Geometry: final body of the model. Coordinates: model frame, mm. A direction names the side the tool comes from. Give positions to 0.01 mm unless a question says otherwise; leave off trailing zeros. Order: outer loops, then holes, each group sorted by start corner. A loop starts at its lowest first (then second) coordinate and runs counter-clockwise, first axis right, second up. Notation, with made-up numbers: (36.25, -31.75) - (84.25, -31.75) arc R19 ccw to (84.25, -23.75) - close; hole circle Ø6 at (-14.5, 5.5). An arc over 180 degrees is marked (long way). Use one line per item in the form item = value.
from build123d import *

# Parameters (mm, degrees)
EXTRUDE_1_DEPTH     = 9
CUT_EXTRUDE_START   = 7.5
CUT_EXTRUDE_1_DEPTH = 142.076331988
CUT_EXTRUDE_START_2 = 8
CUT_EXTRUDE_2_DEPTH = 141.576331988
CUT_EXTRUDE_START_3 = 4.5
CUT_EXTRUDE_3_DEPTH = 145.076331988
CHAMFER_1_SIZE      = 1


# Read off the part's stored shape, not the designer's step: M22 机械螺纹 螺柱1
with BuildPart() as part:
    # 草图1 → 旋转1 (revolve)
    with BuildSketch(Plane.XY, mode=Mode.PRIVATE) as revolve_1_sk:
        Polygon((0, 0), (0, 8.5), (3.9, 8.5), (3.9, 8.1), (5, 8.1), (5, 8.5), (17, 8.5), (17, 12), (34, 12), (34, 17.5), (40, 17.5), (40, 12.5), (55, 12.5), (55, 11), (97, 11), (97, 8.5), (109, 8.5), (109, 7.5), (124, 7.5), (124, 0), align=None)
    revolve(revolve_1_sk.sketch.rotate(Axis((0, 0, 0), (1, 0, 0)), 90), axis=Axis((0, 0, 0), (1, 0, 0)))

    # 草图2 → 凸台-拉伸1 (add)
    with BuildSketch(Plane.ZY.offset(-34)):
        with BuildLine():
            ThreePointArc((1.769346299, -11.868842137), (-12, 0), (1.769346299, 11.868842137))
            ThreePointArc((1.769346299, 11.868842137), (-17.516638735, 20.354713861), (-29.814759189, 37.463643428))
            ThreePointArc((-29.814759189, 37.463643428), (-31.910579937, 39.994896928), (-35.125, 40.678426408))
            ThreePointArc((-35.125, 40.678426408), (-71, 0), (-35.125, -40.678426408))
            ThreePointArc((-35.125, -40.678426408), (-31.910579937, -39.994896928), (-29.814759189, -37.463643428))
            ThreePointArc((-29.814759189, -37.463643428), (-17.516638735, -20.354713861), (1.769346299, -11.868842137))
        make_face()
    extrude(amount=EXTRUDE_1_DEPTH)

    # 草图3 → 切除-拉伸1 (cut, through all)
    with BuildSketch(Plane.XY.offset(CUT_EXTRUDE_START)):
        with BuildLine():
            Line((59, 3), (71, 3))
            ThreePointArc((71, 3), (74, 0), (71, -3))
            Line((71, -3), (59, -3))
            ThreePointArc((59, -3), (56, 0), (59, 3))
        make_face()
    extrude(amount=CUT_EXTRUDE_1_DEPTH, mode=Mode.SUBTRACT)

    # M22 机械螺纹 螺柱1 outline → M22 机械螺纹 螺柱1 (revolve, cut)
    with BuildSketch(Plane.YX):
        Polygon((11, 97), (9.647, 97), (11, 95.647), align=None)
    revolve(axis=Axis((0, 0, 0), (1, 0, 0)), mode=Mode.SUBTRACT)

    # 草图4 → 切除-拉伸2 (cut, through all)
    with BuildSketch(Plane.XY.offset(CUT_EXTRUDE_START_2)):
        with BuildLine():
            Line((81, 2.5), (110.572522736, 2.5))
            ThreePointArc((110.572522736, 2.5), (113.072522736, 0), (110.572522736, -2.5))
            Line((110.572522736, -2.5), (81, -2.5))
            ThreePointArc((81, -2.5), (78.5, 0), (81, 2.5))
        make_face()
    extrude(amount=CUT_EXTRUDE_2_DEPTH, mode=Mode.SUBTRACT)

    # 草图6 → 切除-拉伸3 (cut, through all)
    with BuildSketch(Plane.XY.offset(CUT_EXTRUDE_START_3)):
        with BuildLine():
            Line((111.5, 2.5), (120.5, 2.5))
            ThreePointArc((120.5, 2.5), (123, 0), (120.5, -2.5))
            Line((120.5, -2.5), (111.5, -2.5))
            ThreePointArc((111.5, -2.5), (109, 0), (111.5, 2.5))
        make_face()
    extrude(amount=CUT_EXTRUDE_3_DEPTH, mode=Mode.SUBTRACT)

    # 倒角1
    chamfer_1_edges = [part.edges().sort_by_distance(p)[0] for p in [
        (124, 0, -7.5),
        (0, 0, -8.5),
    ]]
    chamfer(chamfer_1_edges, length=CHAMFER_1_SIZE)


solid = part.part
(1) Ray query, line 1 along X through (y, z) = (12.5, -60); line 2 along Z through (x, y) = (46, 6); line 3 along Y through (x, z) = (57, 8). Return the intervals inside material, ascending.
Computed values:
line_1 = 25 to 34
line_2 = -10.97 to 10.97
line_3 = -7.55 to -2.24, 2.24 to 7.55
(2) Cut plane B-B on y = 19.5. Output: boundary loops of the cut face in (x, z), plus the area to 3 significant figures.
Computed values:
outline = (25, -66.07) - (34, -66.07) - (34, -16.42) - (25, -16.42) - close
area = 447 mm²
(3) Cut plane C-C on x = 21. Output: boundary loops of the cut face in (y, z).
Computed values:
outline = circle Ø24 at (0, 0)
(4) Contact query for flat-ended pins moving along their axis: pin 1 Ø6.5 at (x, y) = (63.5, -1) entering from +Z; pin 2 Ø12 at (x, z) = (106, 4) entering from +Y; pin 3 Ø0.8 at (x, z) = (89, 9) entering from -Y; pin 4 Ø13 at (y, z) = (-5.5, 2.5) entering from -X. Output: stop coordinate, or through.
Computed values:
pin_1 = 10.58
pin_2 = 8.5
pin_3 = -6.86
pin_4 = 0
(5) Reachability of faces 1 (the face through (34, -0.1, 12.2)), 2 (the face through (23.73, 4.596, 11.085)), 3 (the face through (123, 0, 6)), 4 (the face through (97, 4, -8)), 5 (the face through (29.563, -20.544, -17.748)) from +Z, -Z, +X, -X, +Y, -Y: full face, straight path, thin tool, end or side. Return the list, or none.
Computed values:
face_1 = +Z, -X
face_2 = -X
face_3 = +Z
face_4 = +X
face_5 = +Z, -X, -Y
(6) Pull-direction query (Y, two-part tool) for faces 6 (the face through (94, 0, 8)), 7 (the face through (47.605, -3.755, 11.923)), 8 (the face through (17, -8.2, 2.8)); classes: released by +Y, released by -Y, zero draft, split by the parting line, or undercut.
Computed values:
face_6 = undercut
face_7 = split by the parting line
face_8 = zero draft
(7) Cut plane A-A on x = 103. Output: boundary loops of the cut face in (y, z).
Computed values:
outline = (-2.5, 8) - (-2.5, 8.12) arc R8.5 ccw (long way) to (2.5, 8.12) - (2.5, 8) - close
